```python
from build123d import *

# Parameters (mm, degrees)
SKETCH2_W               = 88.5
SKETCH2_H               = 56
BOSS_EXTRUDE1_DEPTH     = 3
SKETCH3_W               = 63.5
SKETCH3_H               = 56
BOSS_EXTRUDE2_DEPTH     = 11
SKETCH4_W               = 22
SKETCH4_H               = 51
BOSS_EXTRUDE3_DEPTH     = 14.5
SKETCH5_W               = 4
SKETCH5_H               = 17
SKETCH5_W_2             = 8
SKETCH5_H_2             = 7.5
SKETCH5_H_3             = 20
CUT_EXTRUDE1_DEPTH      = 4.5
CUT_EXTRUDE1_DEPTH_BACK = 11
SKETCH6_R               = 1.25
CUT_EXTRUDE2_DEPTH      = 18.5
CUT_EXTRUDE2_DEPTH_BACK = 1
SKETCH8_R               = 3
BOSS_EXTRUDE4_DEPTH     = 2.5


with BuildPart() as part:
    # Sketch2 → Boss-Extrude1 (new body)
    with BuildSketch(Plane(origin=(0, 0, 0), x_dir=(1, 0, 0), z_dir=(0, 1, 0))):
        with Locations((44.25, 28)):
            Rectangle(SKETCH2_W, SKETCH2_H)
    extrude(amount=BOSS_EXTRUDE1_DEPTH)

    # Sketch3 → Boss-Extrude2 (add)
    with BuildSketch(Plane(origin=(0, 3, 0), x_dir=(1, 0, 0), z_dir=(0, 1, 0))):
        with Locations((53.75, 28)):
            Rectangle(SKETCH3_W, SKETCH3_H)
    extrude(amount=BOSS_EXTRUDE2_DEPTH)

    # Sketch4 → Boss-Extrude3 (add)
    with BuildSketch(Plane(origin=(0, 3, 0), x_dir=(1, 0, 0), z_dir=(0, 1, 0))):
        with Locations((11, 28)):
            Rectangle(SKETCH4_W, SKETCH4_H)
    extrude(amount=BOSS_EXTRUDE3_DEPTH)

    # Sketch5 → Cut-Extrude1 (cut, two sides)
    with BuildSketch(Plane(origin=(0, 14, 0), x_dir=(1, 0, 0), z_dir=(0, 1, 0))) as cut_extrude1_sk:
        with Locations((83.5, 8.5)):
            Rectangle(SKETCH5_W, SKETCH5_H)
        with Locations((83.5, 47.5)):
            Rectangle(SKETCH5_W, SKETCH5_H)
        with Locations((26, 3.75)):
            Rectangle(SKETCH5_W_2, SKETCH5_H_2)
        with Locations((26, 46)):
            Rectangle(SKETCH5_W_2, SKETCH5_H_3)
    extrude(amount=CUT_EXTRUDE1_DEPTH, mode=Mode.SUBTRACT)
    extrude(cut_extrude1_sk.sketch, amount=-CUT_EXTRUDE1_DEPTH_BACK, mode=Mode.SUBTRACT)

    # Sketch6 → Cut-Extrude2 (cut, two sides)
    with BuildSketch(Plane(origin=(0, 0, 0), x_dir=(1, 0, 0), z_dir=(0, 1, 0))) as cut_extrude2_sk:
        with Locations((84.95, 52.45)):
            Circle(SKETCH6_R)
        with Locations((84.95, 3.55)):
            Circle(SKETCH6_R)
        with Locations((26.55, 3.55)):
            Circle(SKETCH6_R)
        with Locations((26.55, 52.45)):
            Circle(SKETCH6_R)
    extrude(amount=CUT_EXTRUDE2_DEPTH, mode=Mode.SUBTRACT)
    extrude(cut_extrude2_sk.sketch, amount=-CUT_EXTRUDE2_DEPTH_BACK, mode=Mode.SUBTRACT)

    # Sketch8 → Boss-Extrude4 (add)
    with BuildSketch(Plane(origin=(0, 0, -56), x_dir=(-1, 0, 0), z_dir=(0, 0, -1))):
        with Locations((-35, 9.5)):
            Circle(SKETCH8_R)
    extrude(amount=BOSS_EXTRUDE4_DEPTH)


solid = part.part
```
Design review of the part built by this model. Coordinates are the model's own, in mm. A direction names the side the tool comes from. Round coordinates to 2 decimals unless told otherwise and drop trailing zeros. Write each loop counter-clockwise with the first axis right and the second up, starting at its lowest first coordinate (ties: lowest second). Pieces come first, ordered by that corner, then holes.
Item 1: We need section D-D on x = 18. Write out the cut boundary in (y, z).
Item 2: For probe 1 along X at (y, z) = (1.05, -3.55); probe 2 along Z at (x, y) = (84.95, 1.6); probe 3 along X at (y, z) = (4, -43), list the stretches that pass through material, from the lowest coordinate up.
Item 3: We need section B-B on y = 9.5. Write out the cut boundary in (x, z), and give its area (3 significant figures).
Item 4: For faces 1 (the flat face through (22, 15, -33)), 2 (the flat face through (83, 9, -39)), 3 (the flat face through (26, 9, -36)), 4 (the flat face through (11, 10, -2.5)), 5 (the flat face through (11, 10, -53.5)), list the 3-axis set-ups (+Z, -Z, +X, -X, +Y, -Y) from which the entire face can be reached by the end or side of a thin tool; tool diameter is ignored.
Item 5: Clearance check with flat-ended pins moving along their axes: pin 1 Ø6.5 at (x, y) = (26.5, 7.5) entering from -Z; pin 2 Ø6 at (y, z) = (10, -4) entering from -X; pin 3 Ø6 at (x, z) = (48.5, -37.5) entering from +Y; pin 4 Ø4 at (y, z) = (13, -16.5) entering from +X. State where each tip first meets the part, or that it passes through.
Item 6: The part is to be moulded in two halves that separate along X. For faces 6 (the flat face through (83, 9, -17)), 7 (the cylindrical face through (83.7, 1.5, -3.6)), 8 (the flat face through (81.5, 9, -47)), say which applies: +X half, -X half, draft (parallel to the pull), parting line (faces both ways), or undercut.
Item 7: We need section C-C on z = -33.5. Write out the cut boundary in (x, y).
Item 8: We need section A-A on z = -3.55. Write out the cut boundary in (x, y).
Returned:
1. outline: (0, -56) - (3, -56) - (3, -53.5) - (17.5, -53.5) - (17.5, -2.5) - (3, -2.5) - (3, 0) - (0, 0) - close
2. probe 1: x = 0 to 25.3, 27.8 to 83.7, 86.2 to 88.5
2. probe 2: z = -56 to -53.7, -51.2 to -4.8, -2.3 to 0
2. probe 3: x = 0 to 22, 30 to 81.5
3. outline: (0, -53.5) - (22, -53.5) - (22, -36) - (30, -36) - (30, -56) - (32, -56) - (32, -58.5) - (38, -58.5) - (38, -56) - (81.5, -56) - (81.5, -39) - (85.5, -39) - (85.5, -17) - (81.5, -17) - (81.5, 0) - (30, 0) - (30, -7.5) - (22, -7.5) - (22, -2.5) - (0, -2.5) - close
3. area: 4,340 mm2
4. face 1: +Y
4. face 2: -Z, +X, +Y
4. face 3: -Z, +Y
4. face 4: +Z, -X, +Y
4. face 5: -Z, -X, +Y
5. pin 1: stops at z = -36
5. pin 2: stops at x = 0
5. pin 3: stops at y = 14
5. pin 4: stops at x = 85.5
6. face 6: draft
6. face 7: undercut
6. face 8: +X half
7. outline: (0, 0) - (88.5, 0) - (88.5, 3) - (85.5, 3) - (85.5, 14) - (22, 14) - (22, 17.5) - (0, 17.5) - close
8. outline: (0, 0) - (25.3, 0) - (25.3, 3) - (22, 3) - (22, 17.5) - (0, 17.5) - close; (27.8, 0) - (83.7, 0) - (83.7, 3) - (81.5, 3) - (81.5, 14) - (30, 14) - (30, 3) - (27.8, 3) - close; (86.2, 0) - (88.5, 0) - (88.5, 3) - (86.2, 3) - close
